Design review of the part built by this model. Coordinates are the model's own, in mm. Round coordinates to 2 decimals unless told otherwise and drop trailing zeros. Loops run counter-clockwise (first coordinate to the right, second up) from the corner with the lowest first, then second, coordinate; pieces in that order, holes last. Notation, with made-up numbers: M 44,-3 L 90,-3 A28 cw 90,15 Z; hole C -14.5,49 d8. An arc over 180 degrees is marked long. Use a Markdown table: item, result.
from build123d import *

# Parameters (mm, degrees)
SKETCH1_R           = 1.6
BOSS_EXTRUDE1_DEPTH = 5


with BuildPart() as part:
    # Sketch1 → Boss-Extrude1 (new body)
    with BuildSketch(Plane.XY):
        with BuildLine():
            Line((-75, -72.5), (-75, -90.625))
            Line((-75, -90.625), (75, -90.625))
            Line((75, -90.625), (75, -72.5))
            Line((75, -72.5), (60, -72.5))
            Line((60, -72.5), (60, -20))
            Line((60, -20), (75, -20))
            Line((75, -20), (75, 11.191407718))
            add(Edge.make_bspline(
                [(40.797859307, 73.529184669), (29.113413748, 68.584091893), (21.698756749, 49.837173387), (43.872198756, 22.538291001), (75.106478131, 22.355404036), (75, 11.191407718)],
                knots=[0.187825193, 0.187825193, 0.187825193, 0.187825193, 0.468621415, 0.712802941, 1, 1, 1, 1], degree=3))
            ThreePointArc((40.797859307, 73.529184669), (40.890658025, 73.576842128), (40.981293421, 73.628495399))
            ThreePointArc((40.981293421, 73.628495399), (41.118145392, 73.723771319), (41.210746684, 73.862447067))
            ThreePointArc((41.210746684, 73.862447067), (41.223041239, 76.211736408), (39.620297917, 77.929445758))
            ThreePointArc((39.620297917, 77.929445758), (33.882326143, 80.400449206), (27.994286118, 82.488788925))
            ThreePointArc((27.994286118, 82.488788925), (26.19343045, 82.774292897), (24.38900087, 82.512324293))
            ThreePointArc((24.38900087, 82.512324293), (20.964990276, 80.761920244), (18.364057527, 77.929445758))
            ThreePointArc((18.364057527, 77.929445758), (10.722602644, 61.575298771), (11.31305575, 43.533643593))
            ThreePointArc((11.31305575, 43.533643593), (9.427933785, 33.83519482), (0.573242194, 29.452498133))
            Line((0.573242194, 29.452498133), (-0.573242194, 29.452498133))
            ThreePointArc((-0.573242194, 29.452498133), (-9.427933785, 33.83519482), (-11.31305575, 43.533643593))
            ThreePointArc((-11.31305575, 43.533643593), (-10.722602644, 61.575298771), (-18.364057527, 77.929445758))
            ThreePointArc((-18.364057527, 77.929445758), (-18.578745667, 78.220711537), (-18.771416352, 78.526987162))
            ThreePointArc((-18.771416352, 78.526987162), (-21.256426114, 80.976047617), (-24.38900087, 82.512324293))
            ThreePointArc((-24.38900087, 82.512324293), (-26.19343045, 82.774292897), (-27.994286118, 82.488788925))
            ThreePointArc((-27.994286118, 82.488788925), (-33.882326143, 80.400449206), (-39.620297917, 77.929445758))
            ThreePointArc((-39.620297917, 77.929445758), (-41.223041239, 76.211736408), (-41.210746684, 73.862447067))
            ThreePointArc((-41.210746684, 73.862447067), (-41.118145392, 73.723771319), (-40.981293421, 73.628495399))
            add(Edge.make_bspline(
                [(-40.981293421, 73.628495399), (-29.036410535, 68.745777574), (-21.682695552, 49.95343828), (-43.802890071, 22.593157589), (-74.894409224, 22.356830762), (-75, 11.400592909)],
                knots=[0.184913023, 0.184913023, 0.184913023, 0.184913023, 0.468621415, 0.712802941, 0.998195008, 0.998195008, 0.998195008, 0.998195008], degree=3))
            Line((-75, 11.400592909), (-75, 11.191407718))
            Line((-75, 11.191407718), (-75, -20))
            Line((-75, -20), (-60, -20))
            Line((-60, -20), (-60, -72.5))
            Line((-60, -72.5), (-75, -72.5))
        make_face()
        with Locations((-22.052924911, 36.483296004)):
            Circle(SKETCH1_R, mode=Mode.SUBTRACT)
        with Locations((-18.364057527, 56.292076909)):
            Circle(SKETCH1_R, mode=Mode.SUBTRACT)
        with Locations((-26.753522246, 73.691170186)):
            Circle(SKETCH1_R, mode=Mode.SUBTRACT)
        with Locations((22.052924911, 36.483296004)):
            Circle(SKETCH1_R, mode=Mode.SUBTRACT)
        with Locations((18.364057527, 56.292076909)):
            Circle(SKETCH1_R, mode=Mode.SUBTRACT)
        with Locations((26.753522246, 73.691170186)):
            Circle(SKETCH1_R, mode=Mode.SUBTRACT)
    extrude(amount=BOSS_EXTRUDE1_DEPTH)


solid = part.part
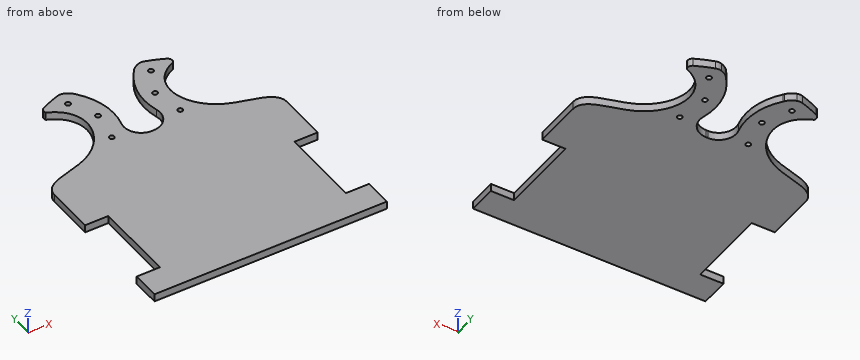
1. Wall thickness on line 1 along X through (y, z) = (-25.5, 4.35); line 2 along Y through (x, z) = (0, 3.1) (1 decimal); line 3 along Y through (x, z) = (32.5, 3.6) (3 decimals): over which ranges is each line inside the solid? List them lowest first. Write a range as from..to.
Check values:
| item | result |
|---|---|
| line 1 | x = -60..60 |
| line 2 | y = -90.6..29.5 |
| line 3 | y = -90.625..38.295, 68.032..80.93 |
2. Take a section at A-A on z = 2.6. Count the separate pieces of the cut face and the enclosed holes in it, and give its area (3 significant figures).
Check values:
| item | result |
|---|---|
| separate pieces | 1 |
| enclosed holes | 6 |
| area | 18,100 mm² |
3. Insertion check: pin 1 (3 mm diameter, centred on y = -46, z = 4.5, fed in from -X); pin 2 (1 mm diameter, centred on y = 57.5, z = 2.5, fed in from -X); pin 3 (3 mm diameter, centred on x = -22.05, y = 36.48, fed in from +Z); pin 4 (1.3 mm diameter, centred on x = 0.5, z = 2, fed in from +Y). Each pin has a flat end and moves straight along its axis. Give the tip position at first contact, or say it passes through.
Check values:
| item | result |
|---|---|
| pin 1 | stops at x = -60 |
| pin 2 | stops at x = -27.13 |
| pin 3 | passes through |
| pin 4 | stops at y = 29.47 |
4. Take a section at B-B on y = -49. Give the boundary of the cut face in (x, z), and give its area (3 significant figures).
Check values:
| item | result |
|---|---|
| outline | M -60,0 L 60,0 L 60,5 L -60,5 Z |
| area | 600 mm² |
